Verification items for the finished model (mm, model axes). Round coordinates to 2 decimals unless told otherwise and drop trailing zeros. Loops run counter-clockwise (first coordinate to the right, second up) from the corner with the lowest first, then second, coordinate; pieces in that order, holes last. Notation, with made-up numbers: (25.5, -20.75) -> (49.5, -20.75) arc R23 ccw to (49.5, 18.25) -> close; hole circle Ø3 at (65.25, -31.5). An arc over 180 degrees is marked (long way). Use CSV: the item, a comma, the result in double quotes. Start each with the question number.
```python
from build123d import *

# Parameters (mm, degrees)
SKETCH_1_W      = 1660
SKETCH_1_H      = 159
EXTRUDE_1_DEPTH = 18
CHAMFER_1_SIZE  = 16
CHAMFER_1_SIZE2 = 11.203320611
CHAMFER_2_SIZE  = 16
CHAMFER_2_SIZE2 = 11.203320611


with BuildPart() as part:
    # 草图1 → 凸台-拉伸1 (new body)
    with BuildSketch(Plane.XY):
        Rectangle(SKETCH_1_W, SKETCH_1_H)
    extrude(amount=EXTRUDE_1_DEPTH)

    # 倒角1
    chamfer_1_edges = [part.edges().sort_by_distance(p)[0] for p in [
        (0, 79.5, 18),
    ]]
    chamfer_1_side = [part.faces().sort_by_distance(p)[0] for p in [
        (0, 79.5, 9),
    ]]
    chamfer(chamfer_1_edges, length=CHAMFER_1_SIZE, length2=CHAMFER_1_SIZE2, reference=chamfer_1_side[0])

    # 倒角2
    chamfer_2_edges = [part.edges().sort_by_distance(p)[0] for p in [
        (0, -79.5, 18),
    ]]
    chamfer_2_side = [part.faces().sort_by_distance(p)[0] for p in [
        (0, -79.5, 9),
    ]]
    chamfer(chamfer_2_edges, length=CHAMFER_2_SIZE, length2=CHAMFER_2_SIZE2, reference=chamfer_2_side[0])


solid = part.part
```
Q1. Thickness scan on L1, parallel to Z at x = 664, y = -72.5; L2, parallel to Y at x = -152, z = 15; L3, parallel to Y at x = -373, z = 14.5. Record the ranges inside material, lowest first. Write a range as from..to.
Q2. Cross-section at A-A (x = 37.5). Record the boundary of the cut face in (y, z).
Q3. Cross-section at B-B (z = 11). Record the boundary of the cut face in (x, y).
Q4. Release check for a two-part mould opening along Z. For faces 1 (the face through (-12, 1, 0)), 2 (the face through (-12, 1, 18)) record: +Z half, -Z half, draft (parallel to the pull), parting line (faces both ways), or undercut.
Q5. Depth check by flat-ended pin: pin 1 Ø5 at (x, z) = (621.5, 9) entering from +Y. Enter the tip coordinate at first touch or a pass-through.
Answer list:
1,L1,"z = 0..12"
1,L2,"y = -70.4..70.4"
1,L3,"y = -70.75..70.75"
2,outline,"(-79.5, 0) -> (79.5, 0) -> (79.5, 2) -> (68.3, 18) -> (-68.3, 18) -> (-79.5, 2) -> close"
3,outline,"(-830, -73.2) -> (830, -73.2) -> (830, 73.2) -> (-830, 73.2) -> close"
4,face 1,"-Z half"
4,face 2,"+Z half"
5,pin 1,"stops at y = 76.35"
